from build123d import *

# Parameters (mm, degrees)
F0_W     = 50.8
F0_H     = 25.4
F1_DEPTH = 50.8
F2_R     = 5.08
F4_D     = 6.35


with BuildPart() as f1:
    # F0 (on Front) → F1 (new body)
    with BuildSketch(Plane.XZ):
        with Locations((25.4, 12.7)):
            Rectangle(F0_W, F0_H)
    extrude(amount=-F1_DEPTH)

    # F2
    f2_edges = [f1.edges().sort_by_distance(p)[0] for p in [
        (50.8, 25.4, 25.4),
        (50.8, 0, 12.7),
        (25.4, 0, 25.4),
    ]]
    fillet(f2_edges, radius=F2_R)

    # F4 (through all)
    with Locations(Plane.XY.offset(25.4)):
        with Locations((25.4, 25.4)):
            Hole(F4_D / 2)


solid = f1.part
Can you work these out from the model? Positions are in its coordinate system, mm. Round coordinates to 2 decimals unless told otherwise and drop trailing zeros. Order: outer loops, then holes, each group sorted by start corner. A loop starts at its lowest first (then second) coordinate and runs counter-clockwise, first axis right, second up. Notation, with made-up numbers: (62.5, -6.75) - (91.5, -6.75) arc R12 cw to (91.5, 16.25) - close; hole circle Ø5 at (80.5, -27). An arc over 180 degrees is marked (long way). Answer in a Markdown table with one row per item.
(1) For P1, Ø2, axis at x = 43.5, y = 14.5, coming from the -Z side; P2, Ø4, axis at x = 25.4, y = 25.4, coming from the -Z side, each with a flat end and sliding along its axis, tell me the tip position at first contact or that it passes through.
From the geometry:
| item | result |
|---|---|
| P1 | stops at z = 0 |
| P2 | passes through |
(2) Suppose I cut it at A-A, the plane x = 25.4. Please give me the cut outline in (y, z) (3 decimals), plus the area to 3 significant figures.
From the geometry:
| item | result |
|---|---|
| outline | (0, 0) - (22.225, 0) - (22.225, 25.4) - (5.08, 25.4) arc R5.08 ccw to (0, 20.32) - close; (28.575, 0) - (50.8, 0) - (50.8, 25.4) - (28.575, 25.4) - close |
| area | 1,120 mm2 |
(3) If we mould it in two halves opening along Y, with no side actions, what happens to faces 1 (the face through (23, 0, 10)), 2 (the face through (31, 25, 0)), 3 (the face through (22.37, 26.35, 12.52))? For each: released by +Y, released by -Y, zero draft, split by the parting line, or undercut.
From the geometry:
| item | result |
|---|---|
| face 1 | released by -Y |
| face 2 | zero draft |
| face 3 | undercut |
(4) Suppose I cut it at B-B, the plane y = 25.4. Please give me the cut outline in (x, z) (3 decimals).
From the geometry:
| item | result |
|---|---|
| outline | (0, 0) - (22.225, 0) - (22.225, 25.4) - (0, 25.4) - close; (28.575, 0) - (50.8, 0) - (50.8, 20.32) arc R5.08 ccw to (45.72, 25.4) - (28.575, 25.4) - close |
(5) Please list where these lines run through material, in increasing order: L1, parallel to Y at x = 25.4, z = 16.25 (3 decimals); L2, parallel to Y at x = 28, z = 17.5; L3, parallel to X at y = 25, z = 23.25. Write a range as from..to.
From the geometry:
| item | result |
|---|---|
| L1 | y = 0..22.225, 28.575..50.8 |
| L2 | y = 0..23.58, 27.22..50.8 |
| L3 | x = 0..22.25, 28.55..49.87 |
